Input: part model. Units: mm. Frame: model coordinates. A direction names the side the tool comes from. Coordinates: 2 decimals unless noted, no trailing zeros. Write each loop counter-clockwise with the first axis right and the second up, starting at its lowest first coordinate (ties: lowest second). Pieces come first, ordered by that corner, then holes. Notation, with made-up numbers: M 39,-21 L 92,-21 A21 cw 92,16 Z; hole C 0.25,-26 d8. An arc over 180 degrees is marked long. Use CSV: the item, a comma, the result in double quotes.
Autodesk Inventor part; units mm, degrees
ref_plane "Work Plane1" through (7.5584, 0, 0) normal (0, 0, -1) x (1, 0, 0)
ref_plane "YZ Plane" through (0, 0, 0) normal (1, 0, 0) x (0, 1, 0)
ref_plane "XZ Plane" through (0, 0, 0) normal (0, 1, 0) x (-1, 0, 0)
sketch "Sketch1" plane through (0, 0, 0) normal (0, 0, 1) x (1, 0, 0)
  line L0 (-11.43, 0) -> (68.58, 0)
  line L1 (0, 0) -> (57.15, 0)
  line L2 (57.15, 0) -> (57.15, 3.175)
  line L3 (57.15, 3.175) -> (5.8928, 3.175)
  line L4 (5.8928, 3.175) -> (4.4826, 3.175)
  line L5 (4.4826, 3.175) -> (2.7178, 3.175)
  line L6 (2.7178, 3.175) -> (2.7178, 4.1584)
  line L7 (2.7178, 4.1584) -> (0.5327, 6.0579)
  line L8 (0.5327, 6.0579) -> (0, 6.0579)
  line L9 (0, 6.0579) -> (0, 0)
  line L10 (0, -1.2116) -> (0, 7.2695)
  line L11 (5.8928, 3.175) -> (2.7178, 3.175) construction
  dimension "d2" = 57.15
  dimension "d3" = 2.7178
  dimension "d4" = 51.2572
  dimension "d5" = 1.4102
  dimension "d6" = 6.35
  dimension "d7" = 6.35
  dimension "d8" = 8.3168
  dimension "d9" = 12.1158
  dimension "d10" = 41
revolve "Body" add sketch "Sketch1" angle 360 about axis through (0, 0, 0) along (1, 0, 0)
sketch "Sketch2" plane through (0, 0, 0) normal (-1, 0, 0) x (0, 0, 1)
  circle A0 centre (0, 0) radius 6.0579
  line L0 (-8.4811, 0) -> (8.4811, 0)
  line L1 (-6.0579, 0) -> (-6.0579, 0.9525)
  line L2 (-6.0579, 0.9525) -> (6.0579, 0.9525)
  line L3 (6.0579, 0) -> (6.0579, 0.9525)
  line L4 (-6.0579, 0) -> (-6.0579, -0.9525)
  line L5 (-6.0579, -0.9525) -> (6.0579, -0.9525)
  line L6 (6.0579, 0) -> (6.0579, -0.9525)
  dimension "d15" = 1.905
extrude "Slot" cut sketch "Sketch2" against normal blind 1.27 contours L0 A0 L2 | L6 L5 A0 | A0 L5 L0 | A0 L2 L3 | L1 L2 A0 | A0 L5 L4
thread "Thread"
ref_plane "Work Plane1" through (7.5584, 0, 0) normal (0, 0, -1) x (1, 0, 0)
equation "\"d2\" = NLG"
equation "\"d3\" = KOH"
equation "\"d4\" = GEL"
equation "\"d5\" = GAL"
equation "\"d6\" = GD"
equation "\"d7\" = BDM"
equation "\"d8\" = KOD1"
equation "\"d9\" = KOD"
equation "\"d10\" = 0.5 * SEWI"
equation "\"d15\" = SBR"
equation "\"d16\" = STI"
equation "\"d12\" = GEL"
equation "\"NND\" = 6.35"
equation "\"NLG\" = 57.15"
equation "\"GEL\" = 51.2572"
equation "\"KOH\" = 2.7178"
equation "\"KOD\" = 12.1158"
equation "\"SBR\" = 1.905"
equation "\"STI\" = 1.27"
equation "\"GAL\" = 1.41021"
equation "\"SPD\" = 4.445"
equation "\"GD\" = NND"
equation "\"KOD1\" = 8.3168"
equation "\"BDM\" = NND"
equation "\"SEWI\" = 82deg"
equation "\"GUL\" = 0.0254"
equation "\"THREADDIA\" = 6.35"
equation "\"TOA\" = 30deg"
equation "\"GD1\" = SPD"
properties part number "ANSI B18.6.3 - 1/4-20 UNC x 2.25, SUFCHMSI" material "Steel, Mild"
1. Access query for faces 1 (the cylindrical face through (29.55, -0.69, 3.1)), 2 (the flat face through (1.27, 0, 0)), 3 (the cylindrical face through (0.263, -6.057, -0.12)). Directions: +Z, -Z, +X, -X, +Y, -Y. A direction counts if a zero-diameter tool reaches every point of the face in a straight line with its end or side. Return the directions, or none.
Resolved:
face 1,"+X"
face 2,"+Z, -Z, -X"
face 3,"+X, -X, -Y"
2. Mould query, pull axis Y, two halves, no side actions, for faces 4 (the cylindrical face through (0.263, 6.057, 0.12)), 5 (the flat face through (1, 0.952, 0)), 6 (the flat face through (2.718, -3, -2)), 7 (the flat face through (1, -0.952, 0)). Classes: pulls with the +Y half, pulls with the -Y half, needs draft (parallel to the pull), parting line crosses it, or undercut.
Resolved:
face 4,"pulls with the +Y half"
face 5,"undercut"
face 6,"needs draft"
face 7,"undercut"
3. Contact query for flat-ended pins moving along their axis: pin 1 Ø1.5 at (y, z) = (2, -3.5) entering from -X; pin 2 Ø1.5 at (y, z) = (4, -4) entering from +X; pin 3 Ø1 at (x, z) = (1, -3) entering from +Y; pin 4 Ø5 at (x, z) = (30.5, 3.5) entering from +Y. Output: stop coordinate, or through.
Resolved:
pin 1,"stops at x = 0"
pin 2,"stops at x = 1.86"
pin 3,"stops at y = 5.36"
pin 4,"stops at y = 3.01"
4. Material intervals for line 1 (Z direction, x = 4, y = -0.25); line 2 (X direction, y = 3.75, z = 0.5), sorted ascending. Write a range as [from, to].
Resolved:
line 1,"z = [-3.17, 3.17]"
line 2,"x = [0, 2.72]"
5. Section B-B (y = 0). Return loops of the section in (x, z) (3 decimals), then the cut area to 3 significant figures.
Resolved:
outline,"M 1.27,-5.417 L 2.718,-4.158 L 2.718,-3.175 L 57.15,-3.175 L 57.15,3.175 L 2.718,3.175 L 2.718,4.158 L 1.27,5.417 Z"
area,"360 mm^2"
6. Section C-C (x = 27). Return loops of the section in (y, z) (3 decimals).
Resolved:
outline,"C 0,0 d6.35"
